Autodesk Inventor part; units mm, degrees
ref_plane "YZ Plane" through (0, 0, 0) normal (1, 0, 0) x (0, 1, 0)
ref_plane "XZ Plane" through (0, 0, 0) normal (0, 1, 0) x (-1, 0, 0)
ref_plane "XY Plane" through (0, 0, 0) normal (0, 0, 1) x (1, 0, 0)
sketch "Sketch1" plane through (0, 0, 0) normal (0, 1, 0) x (-1, 0, 0)
  line L0 (-3, 3) -> (65.9, 3)
  line L1 (65.9, 3) -> (65.9, -90.5)
  line L2 (65.9, -90.5) -> (-3, -90.5)
  line L3 (-3, -90.5) -> (-3, 3)
  circle A0 centre (62.9, 0) radius 1.55
  circle A1 centre (62.9, -87.5) radius 1.55
  circle A2 centre (0, -87.5) radius 1.55
  circle A3 centre (0, 0) radius 1.55
extrude "Extrusion1" add sketch "Sketch1" along normal blind 3
sketch "Sketch2" plane through (0, 3, 0) normal (0, 1, 0) x (1, 0, 0)
  circle A0 centre (0, 0) radius 1.55
  circle A1 centre (0, 87.5) radius 1.55
  circle A2 centre (-62.9, 87.5) radius 1.55
  circle A3 centre (-62.9, 0) radius 1.55
  line L0 (-65.9, -3) -> (3, -3)
  line L1 (3, -3) -> (3, 90.5)
  line L2 (3, 90.5) -> (-65.9, 90.5)
  line L3 (-65.9, 90.5) -> (-65.9, -3)
  line L4 (3, 90.5) -> (-65.9, 90.5)
  circle A4 centre (-46.45, 7) radius 1.35
  circle A5 centre (-46.45, 23) radius 1.35
  circle A6 centre (-16.45, 23) radius 1.35
  circle A7 centre (-16.45, 7) radius 1.35
  circle A8 centre (-16.45, 7) radius 2.5
  circle A9 centre (-16.45, 23) radius 2.5
  circle A10 centre (-46.45, 23) radius 2.5
  circle A11 centre (-46.45, 7) radius 2.5
extrude "Extrusion2" add sketch "Sketch2" along normal blind 3 contours A8 | A9 | A10 | A11
sketch "Sketch3" plane through (0, 3, 0) normal (0, 1, 0) x (1, 0, 0)
  circle A0 centre (-46.45, 23) radius 2.5
  circle A1 centre (-16.45, 7) radius 2.5
  circle A2 centre (-16.45, 23) radius 2.5
  circle A3 centre (-46.45, 7) radius 2.5
  circle A4 centre (0, 0) radius 1.55
  circle A5 centre (0, 87.5) radius 1.55
  circle A6 centre (-62.9, 87.5) radius 1.55
  circle A7 centre (-62.9, 0) radius 1.55
  line L0 (-65.9, -3) -> (3, -3)
  line L1 (3, -3) -> (3, 90.5)
  line L2 (3, 90.5) -> (-65.9, 90.5)
  line L3 (-65.9, 90.5) -> (-65.9, -3)
  circle A8 centre (-46.45, 38) radius 2.5
  circle A9 centre (-46.45, 54) radius 2.5
  circle A10 centre (-16.45, 38) radius 2.5
  circle A11 centre (-16.45, 54) radius 2.5
  circle A12 centre (-46.45, 38) radius 1.35
  circle A13 centre (-46.45, 54) radius 1.35
  circle A14 centre (-16.45, 38) radius 1.35
  circle A15 centre (-16.45, 54) radius 1.35
  dimension "d33" = 5
  dimension "d34" = 5
  dimension "d35" = 5
  dimension "d37" = 15
  dimension "d38" = 15
  dimension "d40" = 16
  dimension "d41" = 2.7
  dimension "d42" = 2.7
  dimension "d44" = 2.7
  dimension "d45" = 2.7
extrude "Extrusion3" add sketch "Sketch3" along normal blind 3 contours A8 | A9 | A10 | A11
sketch "Sketch4" plane through (0, 3, 0) normal (0, 1, 0) x (1, 0, 0)
  circle A0 centre (-16.45, 38) radius 2.5
  circle A1 centre (-46.45, 38) radius 2.5
  circle A2 centre (-46.45, 54) radius 2.5
  circle A3 centre (-16.45, 54) radius 2.5
  circle A4 centre (-46.45, 23) radius 2.5
  circle A5 centre (-16.45, 7) radius 2.5
  circle A6 centre (-16.45, 23) radius 2.5
  circle A7 centre (-46.45, 7) radius 2.5
  circle A8 centre (0, 0) radius 1.55
  circle A9 centre (0, 87.5) radius 1.55
  circle A10 centre (-62.9, 87.5) radius 1.55
  circle A11 centre (-62.9, 0) radius 1.55
  line L0 (-65.9, -3) -> (3, -3)
  line L1 (3, -3) -> (3, 90.5)
  line L2 (3, 90.5) -> (-65.9, 90.5)
  line L3 (-65.9, 90.5) -> (-65.9, -3)
  line L4 (-47.6666, 59.5828) -> (-17.6666, 59.5828)
  line L5 (-17.6666, 59.5828) -> (-17.6666, 70.5828)
  line L6 (-17.6666, 70.5828) -> (-47.6666, 70.5828)
  line L7 (-47.6666, 70.5828) -> (-47.6666, 59.5828)
  line L8 (-47.6666, 73.8193) -> (-17.6666, 73.8193)
  line L9 (-17.6666, 73.8193) -> (-17.6666, 84.8193)
  line L10 (-17.6666, 84.8193) -> (-47.6666, 84.8193)
  line L11 (-47.6666, 84.8193) -> (-47.6666, 73.8193)
  line L12 (-48.6666, 58.5828) -> (-16.6666, 58.5828)
  line L13 (-16.6666, 58.5828) -> (-16.6666, 71.5828)
  line L14 (-16.6666, 71.5828) -> (-48.6666, 71.5828)
  line L15 (-48.6666, 71.5828) -> (-48.6666, 58.5828)
  line L16 (-48.6666, 85.8193) -> (-16.6666, 85.8193)
  line L17 (-16.6666, 85.8193) -> (-16.6666, 72.8193)
  line L18 (-16.6666, 72.8193) -> (-48.6666, 72.8193)
  line L19 (-48.6666, 72.8193) -> (-48.6666, 85.8193)
  dimension "d61" = 32
  dimension "d62" = 13
  dimension "d63" = 32
  dimension "d64" = 13
  dimension "d65" = 1
  dimension "d66" = 30
  dimension "d67" = 0
  dimension "d68" = 1
  dimension "d69" = 30
  dimension "d81" = 11
  dimension "d82" = 11
  dimension "d83" = 1
  dimension "d84" = 1
extrude "Extrusion4" add sketch "Sketch4" along normal blind 3 contours L15 L14 L13 L12 | L16 L17 L18 L19
sketch "Sketch5" plane through (0, 3, 0) normal (0, 1, 0) x (1, 0, 0)
  line L0 (-47.6666, 84.8193) -> (-47.6666, 73.8193)
  line L1 (-47.6666, 73.8193) -> (-17.6666, 73.8193)
  line L2 (-17.6666, 73.8193) -> (-17.6666, 84.8193)
  line L3 (-17.6666, 84.8193) -> (-47.6666, 84.8193)
  line L4 (-47.6666, 70.5828) -> (-47.6666, 59.5828)
  line L5 (-47.6666, 59.5828) -> (-17.6666, 59.5828)
  line L6 (-17.6666, 59.5828) -> (-17.6666, 70.5828)
  line L7 (-17.6666, 70.5828) -> (-47.6666, 70.5828)
  line L8 (-46.6666, 83.8193) -> (-18.6666, 83.8193)
  line L9 (-18.6666, 83.8193) -> (-18.6666, 74.8193)
  line L10 (-18.6666, 74.8193) -> (-46.6666, 74.8193)
  line L11 (-46.6666, 74.8193) -> (-46.6666, 83.8193)
  line L12 (-46.6666, 69.5828) -> (-18.6666, 69.5828)
  line L13 (-18.6666, 69.5828) -> (-18.6666, 60.5828)
  line L14 (-18.6666, 60.5828) -> (-46.6666, 60.5828)
  line L15 (-46.6666, 60.5828) -> (-46.6666, 69.5828)
  point P0 (0, 0)
  dimension "d72" = 1
  dimension "d73" = 1
  dimension "d74" = 1
  dimension "d75" = 1
  dimension "d76" = 1
  dimension "d77" = 1
extrude "Extrusion5" add sketch "Sketch5" along normal blind 2
fillet "Fillet1" radius 3.1 4 edges at (3, 1.5, -90.5) (3, 1.5, 3) (-65.9, 1.5, 3) (-65.9, 1.5, -90.5)
sketch "Sketch6" plane through (0, 3, 0) normal (0, 1, 0) x (1, 0, 0)
  line L0 (-48.6666, 58.5828) -> (-48.6666, 71.5828)
  line L1 (-48.6666, 71.5828) -> (-16.6666, 71.5828)
  line L2 (-16.6666, 71.5828) -> (-16.6666, 58.5828)
  line L3 (-16.6666, 58.5828) -> (-48.6666, 58.5828)
  line L4 (-16.6666, 85.8193) -> (-16.6666, 72.8193)
  line L5 (-16.6666, 72.8193) -> (-48.6666, 72.8193)
  line L6 (-48.6666, 72.8193) -> (-48.6666, 85.8193)
  line L7 (-48.6666, 85.8193) -> (-16.6666, 85.8193)
  circle A0 centre (-16.45, 38) radius 2.5
  circle A1 centre (-46.45, 38) radius 2.5
  circle A2 centre (-46.45, 54) radius 2.5
  circle A3 centre (-16.45, 54) radius 2.5
  circle A4 centre (-46.45, 23) radius 2.5
  circle A5 centre (-16.45, 7) radius 2.5
  circle A6 centre (-16.45, 23) radius 2.5
  circle A7 centre (-46.45, 7) radius 2.5
  circle A8 centre (0, 0) radius 1.55
  circle A9 centre (0, 87.5) radius 1.55
  circle A10 centre (-62.9, 87.5) radius 1.55
  circle A11 centre (-62.9, 0) radius 1.55
  arc A12 (-62.8, 90.5) -> (-65.9, 87.4) centre (-62.8, 87.4) ccw
  line L8 (-65.9, 87.4) -> (-65.9, 0.1)
  arc A13 (-65.9, 0.1) -> (-62.8, -3) centre (-62.8, 0.1) ccw
  line L9 (-62.8, -3) -> (-0.1, -3)
  arc A14 (-0.1, -3) -> (3, 0.1) centre (-0.1, 0.1) ccw
  line L10 (3, 0.1) -> (3, 87.4)
  arc A15 (3, 87.4) -> (-0.1, 90.5) centre (-0.1, 87.4) ccw
  line L11 (-0.1, 90.5) -> (-62.8, 90.5)
  circle A16 centre (-55.95, 3.5059) radius 1.25
  circle A17 centre (-6.95, 3.5059) radius 1.25
  circle A18 centre (-6.95, 61.5059) radius 1.25
  circle A19 centre (-55.95, 61.5059) radius 1.25
  dimension "d85" = 2.5
  dimension "d86" = 2.5
  dimension "d87" = 2.5
  dimension "d88" = 2.5
  dimension "d89" = 49
  dimension "d90" = 49
  dimension "d91" = 58
  dimension "d92" = 9.95
extrude "Extrusion6" cut sketch "Sketch6" against normal blind 10 contours A16 | A17 | A18 | A19
properties part number "Regulator Mount"
Check sheet for the modelled part. Datum: model origin and axes. Units: mm. A direction names the side the tool comes from. Coordinates: 2 decimals unless noted, no trailing zeros. Write each loop counter-clockwise with the first axis right and the second up, starting at its lowest first coordinate (ties: lowest second). Pieces come first, ordered by that corner, then holes. Notation, with made-up numbers: (-15, 4.25) -> (38, 4.25) arc R7 ccw to (38, 16.25) -> close; hole circle Ø8 at (37.25, -26.75). An arc over 180 degrees is marked (long way). Use a Markdown table: item, result.
1. Release check for a two-part mould opening along X. For faces 4 (the cylindrical face through (-56.113, 1.521, -62.745)), 5 (the flat face through (-48.667, 4, -79)), 6 (the flat face through (-15, 6, -53)) record: pulls with the +X half, pulls with the -X half, needs draft (parallel to the pull), parting line crosses it, or undercut.
Reported:
| item | result |
|---|---|
| face 4 | undercut |
| face 5 | pulls with the -X half |
| face 6 | needs draft |
2. Tool access check on faces 1 (the flat face through (-48.667, 4, -65)), 2 (the flat face through (-34, 6, -59)), 3 (the flat face through (-32, 5, -70)). Record the directions out of +Z, -Z, +X, -X, +Y, -Y that give a thin tool (end or side, any length) a straight path to the whole face; none if there is none.
Reported:
| item | result |
|---|---|
| face 1 | -Z, -X, +Y |
| face 2 | +Z, -Z, +X, -X, +Y |
| face 3 | +Y |
3. Sectioned sample at B-B (x = -20). Enter the section's corners in (y, z).
Reported:
| item | result |
|---|---|
| outline | (0, -90.5) -> (3, -90.5) -> (3, -85.82) -> (6, -85.82) -> (6, -84.82) -> (5, -84.82) -> (5, -83.82) -> (3, -83.82) -> (3, -74.82) -> (5, -74.82) -> (5, -73.82) -> (6, -73.82) -> (6, -72.82) -> (3, -72.82) -> (3, -71.58) -> (6, -71.58) -> (6, -70.58) -> (5, -70.58) -> (5, -69.58) -> (3, -69.58) -> (3, -60.58) -> (5, -60.58) -> (5, -59.58) -> (6, -59.58) -> (6, -58.58) -> (3, -58.58) -> (3, 3) -> (0, 3) -> close |
4. Go/stop test with flat-tipped pins: pin 1 Ø1.5 at (x, z) = (-18, -56) entering from -Y; pin 2 Ø0.6 at (y, z) = (3.5, -66) entering from -X; pin 3 Ø3.5 at (x, z) = (-34, -66.5) entering from +Y; pin 4 Ø10 at (x, z) = (-34.5, -79.5) entering from +Y. Record where each tip stops, or that it passes through.
Reported:
| item | result |
|---|---|
| pin 1 | stops at y = 0 |
| pin 2 | stops at x = -48.67 |
| pin 3 | stops at y = 3 |
| pin 4 | stops at y = 5 |
5. Sectioned sample at A-A (x = -6.95). Enter the section's corners in (y, z), plus the area to 4 significant figures.
Reported:
| item | result |
|---|---|
| outline | (0, -90.5) -> (3, -90.5) -> (3, -62.76) -> (0, -62.76) -> close; (0, -60.26) -> (3, -60.26) -> (3, -4.76) -> (0, -4.76) -> close; (0, -2.26) -> (3, -2.26) -> (3, 3) -> (0, 3) -> close |
| area | 265.5 mm2 |
6. Sectioned sample at D-D (z = -34). Enter the section's corners in (x, y).
Reported:
| item | result |
|---|---|
| outline | (-65.9, 0) -> (3, 0) -> (3, 3) -> (-65.9, 3) -> close |
7. Scan lines: line 1 along Z through (x, y) = (-27.5, 3.3); line 2 along X through (y, z) = (3.9, -54); line 3 along X through (y, z) = (1.45, -87.5). Record each from-to range of solid material in increasing order.
Reported:
| item | result |
|---|---|
| line 1 | z = -85.82 to -83.82, -74.82 to -72.82, -71.58 to -69.58, -60.58 to -58.58 |
| line 2 | x = -48.95 to -47.8, -45.1 to -43.95, -18.95 to -17.8, -15.1 to -13.95 |
| line 3 | x = -65.9 to -64.45, -61.35 to -1.55, 1.55 to 3 |
8. Sectioned sample at C-C (z = -23). Enter the section's corners in (x, y).
Reported:
| item | result |
|---|---|
| outline | (-65.9, 0) -> (3, 0) -> (3, 3) -> (-13.95, 3) -> (-13.95, 6) -> (-15.1, 6) -> (-15.1, 3) -> (-17.8, 3) -> (-17.8, 6) -> (-18.95, 6) -> (-18.95, 3) -> (-43.95, 3) -> (-43.95, 6) -> (-45.1, 6) -> (-45.1, 3) -> (-47.8, 3) -> (-47.8, 6) -> (-48.95, 6) -> (-48.95, 3) -> (-65.9, 3) -> close |
